Can you work these out from the model? Positions are in its coordinate system, mm. A direction names the side the tool comes from. Give positions to 0.01 mm unless a question says otherwise; leave off trailing zeros. Order: outer loops, then holes, each group sorted by start corner. A loop starts at its lowest first (then second) coordinate and runs counter-clockwise, first axis right, second up.
Item 1: I want a section at C-C, the plane x = 31. Write out the boundary of the cut face in (y, z).
Item 2: I want a section at A-A, the plane z = 28. Write out the boundary of the cut face in (x, y), then the cut area to 3 significant figures.
Item 3: I want a section at B-B, the plane z = 4.5. Write out the boundary of the cut face in (x, y), then the cut area to 3 significant figures.
Item 4: If I drill on line 1 along Y through (x, z) = (84, 0.8); line 2 along Y through (x, z) = (4, 30.5); line 3 along Y through (x, z) = (44.5, 19), over which ranges is the centre line in solid material (lowest first)?
Item 5: I want a section at D-D, the plane y = 59. Write out the boundary of the cut face in (x, z), then the cut area to 3 significant figures.
Item 6: Which directions (+Z, -Z, +X, -X, +Y, -Y) give clear straight access to the entire face, cutting with the end or side of a thin tool? Please do faces 1 (the flat face through (4, 0, 30)), 2 (the cylindrical face through (88.56, 42.4, 0.39)), 3 (the flat face through (0, 4, 30)), 4 (the flat face through (101, 68, 19)).
Item 7: If we mould it in two halves opening along X, with no side actions, what happens to faces 5 (the cylindrical face through (6.859, 63.203, 19.342)), 6 (the flat face through (110.6, 35, 11)), 7 (the flat face through (106, 2, 38))? For each: +X half, -X half, draft (parallel to the pull), parting line (faces both ways), or undercut.
Item 8: I'm going to push flat-ended pins straight in: pin 1 Ø2.5 at (y, z) = (68, 31) entering from -X; pin 2 Ø6.5 at (x, z) = (4, 32) entering from +Y; pin 3 Ø21 at (x, y) = (61.5, 44) entering from +Z. Where does each tip first touch, or does it pass through?
Autodesk Inventor part; units mm, degrees
ref_plane "rovina_napajeni_znacka2" through (-1.1, 15.7, 13.2) normal (-1, 0, 0) x (0, 0, 1)
ref_plane "YZ Plane" through (0, 0, 0) normal (1, 0, 0) x (0, 1, 0)
ref_plane "XZ Plane" through (0, 0, 0) normal (0, 1, 0) x (-1, 0, 0)
sketch "zakladna" plane through (0, 0, 0) normal (0, 0, 1) x (1, 0, 0)
  line L0 (0, 0) -> (109, 0)
  line L1 (109, 0) -> (109, 70)
  line L2 (109, 70) -> (0, 70)
  line L3 (0, 70) -> (0, 0)
  dimension "d0" = 109
  dimension "d1" = 70
extrude "Extrusion1" add sketch "zakladna" along normal blind 1.2 and the other way blind 0.4
sketch "stena_RJ45" plane through (0, 0, -0.4) normal (0, 0, -1) x (-1, 0, 0)
  line L0 (1.6, 15.7) -> (0, 15.7)
  line L1 (0, 15.7) -> (0, 32.5)
  line L2 (0, 32.5) -> (1.6, 32.5)
  line L3 (1.6, 32.5) -> (1.6, 15.7)
  line L4 (-109, 0) -> (0, 0)
  line L5 (0, 0) -> (0, 70)
  dimension "d4" = 1.6
  dimension "d5" = 16.8
  dimension "d6" = 15.7
  dimension "d7" = 0
sketch "diry_tlacirka_LED" plane through (0, 0, -0.4) normal (0, 0, -1) x (-1, 0, 0)
  line L0 (-109, 70) -> (-109, 0)
  line L1 (-109, 0) -> (-109, 70)
  line L2 (-109, 35) -> (-3.6376, 35)
  line L3 (1.6, 32.5) -> (1.6, 15.7)
  circle A0 centre (-84, 24.1) radius 5.75
  circle A1 centre (-84, 45.9) radius 5.75
  circle A2 centre (-31, 35) radius 3.85
  line L4 (0, 0) -> (0, 70)
  dimension "d9" = 11.5
  dimension "d10" = 7.7
  dimension "d11" = 31
  dimension "d53" = 25
extrude "Extrusion2" cut sketch "diry_tlacirka_LED" against normal blind 2
sketch "steny" plane through (0, 0, -0.4) normal (0, 0, -1) x (-1, 0, 0)
  line L0 (-109, 70) -> (0, 70)
  line L1 (0, 0) -> (-109, 0)
  line L2 (0, 15.7) -> (0, 0)
  line L3 (-109, 0) -> (-109, 70)
  line L4 (0, 0) -> (-109, 0)
  line L5 (-109, 0) -> (-109, 70)
  line L6 (-109, 70) -> (0, 70)
  line L7 (0, 70) -> (0, 32.5)
  line L8 (1.6, 15.7) -> (1.6, -1.6)
  line L9 (1.6, -1.6) -> (-110.6, -1.6)
  line L10 (-110.6, -1.6) -> (-110.6, 71.6)
  line L11 (-110.6, 71.6) -> (1.6, 71.6)
  line L12 (1.6, 71.6) -> (1.6, 32.5)
  line L13 (1.6, 15.7) -> (0, 15.7)
  line L14 (0, 32.5) -> (1.6, 32.5)
  dimension "d42" = 1.6
extrude "Extrusion3" add sketch "steny" against normal blind 23.4
extrude "Extrusion4" add sketch "stena_RJ45" against normal blind 13.6
sketch "Sketch5" plane through (0, 0, 1.2) normal (0, 0, 1) x (1, 0, 0)
  arc A0 (4, 62) -> (8, 66) centre (4, 66) ccw
  line L0 (4, 62) -> (0, 62)
  line L1 (8, 66) -> (8, 70)
  line L2 (0, 70) -> (0, 0)
  line L3 (0, 62) -> (0, 70)
  line L4 (0, 70) -> (8, 70)
  arc A1 (8, 4) -> (4, 8) centre (4, 4) ccw
  line L5 (4, 8) -> (0, 8)
  line L6 (8, 4) -> (8, 0)
  line L7 (0, 8) -> (0, 0)
  line L8 (0, 0) -> (8, 0)
  line L9 (109, 0) -> (0, 0)
  line L10 (0, 0) -> (8, 0)
  line L11 (109, 70) -> (109, 0)
  line L12 (105, 62) -> (109, 62)
  arc A2 (101, 66) -> (105, 62) centre (105, 66) ccw
  line L13 (109, 62) -> (109, 70)
  line L14 (109, 70) -> (101, 70)
  line L15 (101, 66) -> (101, 70)
  line L16 (109, 0) -> (101, 0)
  line L17 (109, 0) -> (101, 0)
  line L18 (101, 4) -> (101, 0)
  line L19 (105, 8) -> (109, 8)
  line L20 (109, 8) -> (109, 0)
  arc A3 (105, 8) -> (101, 4) centre (105, 4) ccw
  point P0 (0, 32.5)
  dimension "d22" = 8
extrude "Extrusion5" add sketch "Sketch5" along normal blind 36.8
sketch "diry_zavitova_vlozka" plane through (0, 0, 38) normal (0, 0, 1) x (1, 0, 0)
  arc A0 (8, 4) -> (4, 8) centre (4, 4) ccw
  arc A1 (4, 62) -> (8, 66) centre (4, 66) ccw
  arc A2 (105, 8) -> (101, 4) centre (105, 4) ccw
  arc A3 (101, 66) -> (105, 62) centre (105, 66) ccw
  point P0 (0, 0)
hole "Hole1" at (105, 4, 38) at (105, 66, 38) at (4, 4, 38) at (4, 66, 38) direction (0, 0, -1) diameter 3.3 depth 12 countersink diameter 3.75 countersink angle 10
fillet "Fillet1" radius 2 4 edges at (-1.6, 71.6, 11.3) (-1.6, -1.6, 11.3) (110.6, -1.6, 11.3) (110.6, 71.6, 11.3)
sketch "znacka_napajeni1" plane through (-1.6, 15.7, 13.2) normal (-1, 0, 0) x (0, 0, 1)
  circle A0 centre (-1, 34.8) radius 0.4
  line L0 (0, 16.8) -> (0, 0)
  line L1 (0, 16.8) -> (9.8, 16.8)
  dimension "d44" = 0.8
  dimension "d45" = 1
  dimension "d46" = 18
ref_plane "rovina_napajeni_znacka2" through (-1.1, 15.7, 13.2) normal (-1, 0, 0) x (0, 0, 1)
sketch "napajeni_znacka2" plane through (-1.1, 15.7, 13.2) normal (-1, 0, 0) x (0, 0, 1)
  point P0 (-13.2, -15.7)
  point P1 (-1, 34.8)
loft "Loft1" cut profiles "znacka_napajeni1" section 2 point at (-1.1, 50.5, 12.2)
properties part number "case_top"
Results list:
1. outline: (-1.6, -0.4) - (31.15, -0.4) - (31.15, 1.2) - (0, 1.2) - (0, 23) - (-1.6, 23) - close; (38.85, -0.4) - (71.6, -0.4) - (71.6, 23) - (70, 23) - (70, 1.2) - (38.85, 1.2) - close
2. outline: (0, 0) - (8, 0) - (8, 4) arc R4 ccw to (4, 8) - (0, 8) - close; (0, 62) - (4, 62) arc R4 ccw to (8, 66) - (8, 70) - (0, 70) - close; (101, 0) - (109, 0) - (109, 8) - (105, 8) arc R4 ccw to (101, 4) - close; (101, 66) arc R4 ccw to (105, 62) - (109, 62) - (109, 70) - (101, 70) - close; hole circle Ø3.3 at (4, 4); hole circle Ø3.3 at (4, 66); hole circle Ø3.3 at (105, 4); hole circle Ø3.3 at (105, 66)
2. area: 208 mm2
3. outline: (-1.6, 0.4) arc R2 ccw to (0.4, -1.6) - (108.6, -1.6) arc R2 ccw to (110.6, 0.4) - (110.6, 69.6) arc R2 ccw to (108.6, 71.6) - (0.4, 71.6) arc R2 ccw to (-1.6, 69.6) - close; hole (0, 8) - (4, 8) arc R4 cw to (8, 4) - (8, 0) - (101, 0) - (101, 4) arc R4 cw to (105, 8) - (109, 8) - (109, 62) - (105, 62) arc R4 cw to (101, 66) - (101, 70) - (8, 70) - (8, 66) arc R4 cw to (4, 62) - (0, 62) - close
3. area: 822 mm2
4. line 1: y = -1.6 to 18.35, 29.85 to 40.15, 51.65 to 71.6
4. line 2: y = 0 to 2.35, 5.65 to 8, 62 to 64.35, 67.65 to 70
4. line 3: y = -1.6 to 0, 70 to 71.6
5. outline: (-1.6, -0.4) - (110.6, -0.4) - (110.6, 23) - (109, 23) - (109, 1.2) - (0, 1.2) - (0, 23) - (-1.6, 23) - close
5. area: 249 mm2
6. face 1: +Z, +X, -X, -Y
6. face 2: +Z, -Z
6. face 3: +Z, -X, +Y, -Y
6. face 4: +Z
7. face 5: undercut
7. face 6: +X half
7. face 7: draft
8. pin 1: stops at x = 0
8. pin 2: stops at y = 70
8. pin 3: stops at z = 1.2
